The listing builds one solid part. Answer for the finished solid, in the listing's coordinates (mm). A direction names the side the tool comes from. Coordinates: 2 decimals unless noted, no trailing zeros. Write each loop counter-clockwise with the first axis right and the second up, starting at its lowest first coordinate (ties: lowest second). Pieces come first, ordered by that corner, then holes. Notation, with made-up numbers: M 44.5,13.5 L 101.5,13.5 A8 cw 101.5,25.5 Z; hole C 83,80 d11. An arc over 180 degrees is marked long. Answer as a JSON object with one key per item and string values. Group by question number.
from build123d import *

# Parameters (mm, degrees)
EXTRUDE_1_DEPTH          = 50
CHAMFER_1_SIZE           = 5
CUT_EXTRUDE_1_DEPTH      = 88.183714076
CUT_EXTRUDE_1_DEPTH_BACK = 88.183714076
SKETCH_2_R               = 15.04
SKETCH_2_R_2             = 2.25
CUT_EXTRUDE_2_DEPTH      = 88.252507127
CUT_EXTRUDE_2_DEPTH_BACK = 88.252507127


with BuildPart() as part:
    # 草图1 → 凸台-拉伸1 (new body)
    with BuildSketch(Plane.XY):
        Polygon((0, 0), (53, 0), (53, 3), (3, 3), (3, 51), (0, 51), align=None)
    extrude(amount=EXTRUDE_1_DEPTH)

    # 倒角1
    chamfer_1_edges = [part.edges().sort_by_distance(p)[0] for p in [
        (53, 1.5, 50),
        (1.5, 51, 50),
        (1.5, 51, 0),
        (53, 1.5, 0),
    ]]
    chamfer(chamfer_1_edges, length=CHAMFER_1_SIZE)

    # 草图2 → 切除-拉伸1 (cut, two sides: drawn at the far end of the back side and taken through both)
    with BuildSketch(Plane(origin=(3, 0, 0), x_dir=(0, 0, -1), z_dir=(1, 0, 0)).offset(-CUT_EXTRUDE_1_DEPTH_BACK)):
        with Locations(Location((-25, 30, 0), (0, 0, 90))):
            Circle(SKETCH_2_R)
        with Locations(Location((-8.735, 46.265, 0), (0, 0, 90))):
            Circle(SKETCH_2_R_2)
        with Locations(Location((-41.265, 46.265, 0), (0, 0, 90))):
            Circle(SKETCH_2_R_2)
        with Locations(Location((-8.735, 13.735, 0), (0, 0, 90))):
            Circle(SKETCH_2_R_2)
        with Locations(Location((-41.265, 13.735, 0), (0, 0, 90))):
            Circle(SKETCH_2_R_2)
    extrude(amount=CUT_EXTRUDE_1_DEPTH + CUT_EXTRUDE_1_DEPTH_BACK, mode=Mode.SUBTRACT)

    # 草图4 → 切除-拉伸2 (cut, two sides: drawn at the far end of the back side and taken through both)
    with BuildSketch(Plane(origin=(0, 3, 0), x_dir=(1, 0, 0), z_dir=(0, 1, 0)).offset(-CUT_EXTRUDE_2_DEPTH_BACK)):
        with BuildLine():
            Line((12, -12), (42, -12))
            ThreePointArc((42, -12), (44, -10), (42, -8))
            Line((42, -8), (12, -8))
            ThreePointArc((12, -8), (10, -10), (12, -12))
        make_face()
        with BuildLine():
            Line((12, -38), (42, -38))
            ThreePointArc((42, -38), (44, -40), (42, -42))
            Line((42, -42), (12, -42))
            ThreePointArc((12, -42), (10, -40), (12, -38))
        make_face()
    extrude(amount=CUT_EXTRUDE_2_DEPTH + CUT_EXTRUDE_2_DEPTH_BACK, mode=Mode.SUBTRACT)


solid = part.part
Item 1: A cutting plane is placed at B-B, the plane z = 25. Write down the section's boundary in (x, y).
Item 2: A tool of negligible diameter and unlimited length cuts with its end or side. For faces 5 (the face through (3, 16, 19)), 6 (the face through (1.479, 44.479, 39.896)), 7 (the face through (27, 1, 8)), from which of +Z, -Z, +X, -X, +Y, -Y can it reach the whole face along a straight path? Write none if from no direction.
Item 3: A cutting plane is placed at A-A, the plane x = 26. Write down the section's boundary in (y, z).
Item 4: For a pull along Y with two mould halves and no side action, classify faces 1 (the face through (1.48, 28.04, 39.91)), 2 (the face through (2, 48, 2)), 3 (the face through (1.48, 15.81, 7.87)), 4 (the face through (27, 1, 42)) as +Y half, -Y half, draft (parallel to the pull), parting line (faces both ways), or undercut.
Item 5: A cutting plane is placed at C-C, the plane y = 30. Write down the section's boundary in (x, z), and give its area (3 significant figures).
Item 6: A cutting plane is placed at D-D, the plane y = 12.5. Write down the section's boundary in (x, z).
Item 7: Flat-ended cylindrical pins translate along their axes: pin 1 Ø15 at (x, z) = (30.5, 16) entering from +Y; pin 2 Ø4 at (y, z) = (9, 16) entering from -X; pin 3 Ø5 at (y, z) = (46.265, 41.265) entering from +X. Find the tip coordinate at first contact, or state that the pin passes through.
Item 8: Consider L1, parallel to Y at x = 2.05, z = 25; L2, parallel to Y at x = 24, z = 32. Determine where each line is inside the solid, lowest interval first. Write a range as from..to.
Answer:
{
 "1": {"outline": "M 0,0 L 53,0 L 53,3 L 3,3 L 3,14.96 L 0,14.96 Z; M 0,45.04 L 3,45.04 L 3,51 L 0,51 Z"},
 "2": {"face 5": "+Z, -Z, +X, +Y", "face 6": "+X, -X", "face 7": "+Y, -Y"},
 "3": {"outline": "M 0,0 L 3,0 L 3,8 L 0,8 Z; M 0,12 L 3,12 L 3,38 L 0,38 Z; M 0,42 L 3,42 L 3,50 L 0,50 Z"},
 "4": {"face 1": "undercut", "face 2": "+Y half", "face 3": "undercut", "face 4": "draft"},
 "5": {"outline": "M 0,0 L 3,0 L 3,9.96 L 0,9.96 Z; M 0,40.04 L 3,40.04 L 3,50 L 0,50 Z", "area": "59.8 mm2"},
 "6": {"outline": "M 0,0 L 3,0 L 3,6.85 L 0,6.85 Z; M 0,10.62 L 3,10.62 L 3,39.38 L 0,39.38 Z; M 0,43.15 L 3,43.15 L 3,50 L 0,50 Z"},
 "7": {"pin 1": "y = 3", "pin 2": "x = 0", "pin 3": "x = 3"},
 "8": {"L1": "0..14.96, 45.04..51", "L2": "0..3"}
}
